The model under review builds one solid part; all positions refer to its coordinate system, in mm. Face numbers are marked on the shaded views. Coordinates: 2 decimals unless noted, no trailing zeros. Write each loop counter-clockwise with the first axis right and the second up, starting at its lowest first coordinate (ties: lowest second). Pieces come first, ordered by that corner, then holes.
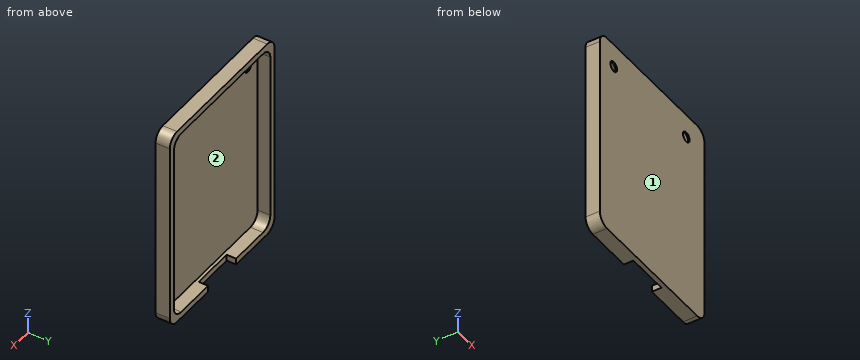
```python
from build123d import *

# Parameters (mm, degrees)
BOSS_EXTRUDE1_DEPTH = 4.5
CUT_EXTRUDE1_DEPTH  = 4
SKETCH3_W           = 13.5
SKETCH3_H           = 6
CUT_EXTRUDE3_DEPTH  = 15
SKETCH4_R           = 1.6
CUT_EXTRUDE4_DEPTH  = 40


with BuildPart() as part:
    # Sketch1 → Boss-Extrude1 (new body)
    with BuildSketch(Plane(origin=(0, 0, 0), x_dir=(1, 0, 0), z_dir=(0, 1, 0))):
        with BuildLine():
            Line((3.5, 0), (47, 0))
            ThreePointArc((47, 0), (49.474873734, 1.025126266), (50.5, 3.5))
            Line((50.5, 3.5), (50.5, 61.5))
            ThreePointArc((50.5, 61.5), (49.474873734, 63.974873734), (47, 65))
            Line((47, 65), (3.5, 65))
            ThreePointArc((3.5, 65), (1.025126266, 63.974873734), (0, 61.5))
            Line((0, 61.5), (0, 3.5))
            ThreePointArc((0, 3.5), (1.025126266, 1.025126266), (3.5, 0))
        make_face()
    extrude(amount=BOSS_EXTRUDE1_DEPTH)

    # Sketch2 → Cut-Extrude1 (cut)
    with BuildSketch(Plane(origin=(0, 4.5, 0), x_dir=(1, 0, 0), z_dir=(0, 1, 0))):
        with BuildLine():
            Line((5.5, 2), (45, 2))
            ThreePointArc((45, 2), (47.474873734, 3.025126266), (48.5, 5.5))
            Line((48.5, 5.5), (48.5, 59.5))
            ThreePointArc((48.5, 59.5), (47.474873734, 61.974873734), (45, 63))
            Line((45, 63), (5.5, 63))
            ThreePointArc((5.5, 63), (3.025126266, 61.974873734), (2, 59.5))
            Line((2, 59.5), (2, 5.5))
            ThreePointArc((2, 5.5), (3.025126266, 3.025126266), (5.5, 2))
        make_face()
    extrude(amount=-CUT_EXTRUDE1_DEPTH, mode=Mode.SUBTRACT)

    # Sketch3 → Cut-Extrude3 (cut)
    with BuildSketch(Plane(origin=(0, 0, -65), x_dir=(-1, 0, 0), z_dir=(0, 0, -1))):
        with Locations((-25.25, 4.5)):
            Rectangle(SKETCH3_W, SKETCH3_H)
    extrude(amount=-CUT_EXTRUDE3_DEPTH, mode=Mode.SUBTRACT)

    # Sketch4 → Cut-Extrude4 (cut)
    with BuildSketch(Plane(origin=(0, 0.5, 0), x_dir=(1, 0, 0), z_dir=(0, 1, 0))):
        with Locations(Location((6.724572176, 7.5, 0), (0, 0, 270))):
            Circle(SKETCH4_R)
        with Locations(Location((41.724572176, 7.5, 0), (0, 0, 270))):
            Circle(SKETCH4_R)
    extrude(amount=-CUT_EXTRUDE4_DEPTH, mode=Mode.SUBTRACT)


solid = part.part
```
Item 1: Take a section at C-C, the plane y = 3.1. Write out the cut boundary in (x, z), plus the area to 3 significant figures.
Solved:
outline: (0, -61.5) arc R3.5 ccw to (3.5, -65) - (18.5, -65) - (18.5, -63) - (5.5, -63) arc R3.5 cw to (2, -59.5) - (2, -5.5) arc R3.5 cw to (5.5, -2) - (45, -2) arc R3.5 cw to (48.5, -5.5) - (48.5, -59.5) arc R3.5 cw to (45, -63) - (32, -63) - (32, -65) - (47, -65) arc R3.5 ccw to (50.5, -61.5) - (50.5, -3.5) arc R3.5 ccw to (47, 0) - (3.5, 0) arc R3.5 ccw to (0, -3.5) - close
area: 419 mm2
Item 2: Take a section at A-A, the plane z = -7.5. Write out the cut boundary in (x, y).
Solved:
outline: (0, 0) - (5.12, 0) - (5.12, 0.5) - (2, 0.5) - (2, 4.5) - (0, 4.5) - close; (8.32, 0) - (40.12, 0) - (40.12, 0.5) - (8.32, 0.5) - close; (43.32, 0) - (50.5, 0) - (50.5, 4.5) - (48.5, 4.5) - (48.5, 0.5) - (43.32, 0.5) - close
Item 3: Take a section at D-D, the plane x = 28.5. Write out the cut boundary in (y, z), plus the area to 3 significant figures.
Solved:
outline: (0, -65) - (1.5, -65) - (1.5, -63) - (0.5, -63) - (0.5, -2) - (4.5, -2) - (4.5, 0) - (0, 0) - close
area: 42.5 mm2
Item 4: Mouldability with a two-part tool opening along Z and no side actions: class the marked faces 1 and 2 as pulls with the +Z half, pulls with the -Z half, needs draft (parallel to the pull), parting line crosses it, or undercut.
Solved:
face 1: needs draft
face 2: undercut
Item 5: To check wall thickness, follow line 1 along X through (y, z) = (0.25, -7.5); line 2 along Z through (x, y) = (15, 2.25); line 3 along X through (y, z) = (0.6, -26). State the ranges of each line that lie inside material, in increasing order.
Solved:
line 1: x = 0 to 5.12, 8.32 to 40.12, 43.32 to 50.5
line 2: z = -65 to -63, -2 to 0
line 3: x = 0 to 2, 48.5 to 50.5
Item 6: Take a section at B-B, the plane x = 7.5. Write out the cut boundary in (y, z).
Solved:
outline: (0, -65) - (4.5, -65) - (4.5, -63) - (0.5, -63) - (0.5, -8.9) - (0, -8.9) - close; (0, -6.1) - (0.5, -6.1) - (0.5, -2) - (4.5, -2) - (4.5, 0) - (0, 0) - close
Item 7: For pin 1 (5 mm diameter, centred on x = 19.5, z = -6.5, fed in from +Y); pin 2 (1 mm diameter, centred on y = 2.5, z = -64, fed in from +X); pin 3 (1 mm diameter, centred on y = 3.5, z = -64.5, fed in from -X), all flat-tipped, find the tip position at first contact; note any pin that passes through.
Solved:
pin 1: stops at y = 0.5
pin 2: stops at x = 49.87
pin 3: stops at x = 1.05
